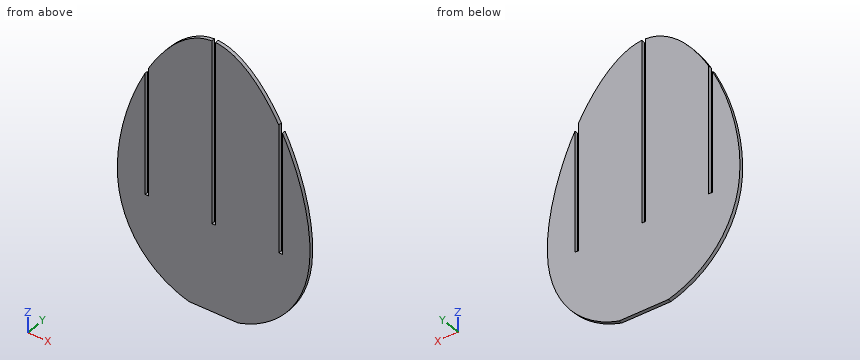
```python
from build123d import *

# Parameters (mm, degrees)
F1_DEPTH = 3


# Not quite as in the source:
# - a feature names something its author has since deleted; it is built from what else it names


with BuildPart() as f1:
    # F0 (on Front) → F1 (new body)
    with BuildSketch(Plane.XZ):
        with BuildLine():
            Line((-95.6991912493, -140.1659290001), (-95.6991912493, 9.7979199733))
            add(Edge.make_bspline(
                [(-95.6991912493, 9.7979199733), (-114.9403248651, 8.8727934734), (-134.0676037648, -9.7150772734), (-148.6991912496, -35.2231978093)],
                knots=[0.0032045269, 0.0032045269, 0.0032045269, 0.0032045269, 0.1265346274, 0.1265346274, 0.1265346274, 0.1265346274], degree=3))
            Line((-148.6991912496, -35.2231978093), (-148.6991912415, -140.1659290001))
            Line((-148.6991912415, -140.1659290001), (-151.6991912415, -140.1659290001))
            Line((-151.6991912415, -140.1659290001), (-151.6991912492, -40.6684138407))
            add(Edge.make_bspline(
                [(-151.6991912492, -40.6684138407), (-167.8134864464, -71.1210787155), (-189.9683027369, -159.0658708259), (-144.3602498784, -204.2889070632), (-114.8366912492, -212.3738275092)],
                knots=[0.135152904, 0.135152904, 0.135152904, 0.135152904, 0.2772924741, 0.4585993514, 0.4585993514, 0.4585993514, 0.4585993514], degree=3))
            Line((-114.8366912492, -212.3738275092), (-73.5616912492, -212.3738275092))
            add(Edge.make_bspline(
                [(-73.5616912492, -212.3738275092), (-44.03813262, -204.2889070632), (1.5699202449, -159.0658708196), (-20.5848960581, -71.1210786912), (-36.6991912644, -40.6684138119)],
                knots=[0.5414006486, 0.5414006486, 0.5414006486, 0.5414006486, 0.7227075259, 0.8648470961, 0.8648470961, 0.8648470961, 0.8648470961], degree=3))
            Line((-36.6991912644, -40.6684138119), (-36.6991912645, -140.1659290001))
            Line((-36.6991912645, -140.1659290001), (-39.6991912645, -140.1659290001))
            Line((-39.6991912645, -140.1659290001), (-39.6991912644, -35.223197782))
            add(Edge.make_bspline(
                [(-39.6991912644, -35.223197782), (-54.3307787472, -9.71507726), (-73.4580576403, 8.8727934739), (-92.6991912493, 9.7979199734)],
                knots=[0.8734653727, 0.8734653727, 0.8734653727, 0.8734653727, 0.9967954731, 0.9967954731, 0.9967954731, 0.9967954731], degree=3))
            Line((-92.6991912493, 9.7979199734), (-92.6991912493, -140.1659290001))
            Line((-92.6991912493, -140.1659290001), (-95.6991912493, -140.1659290001))
        make_face()
    extrude(amount=F1_DEPTH)


solid = f1.part
```
Source: CAD feature listing. Evaluate the final solid. Frame: model axes, mm. Coordinates: 2 decimals unless noted, no trailing zeros. Write each loop counter-clockwise with the first axis right and the second up, starting at its lowest first coordinate (ties: lowest second). Pieces come first, ordered by that corner, then holes. Notation, with made-up numbers: (70, 85.5) - (80, 85.5) arc R21 cw to (80, 115.5) - close; hole circle Ø1 at (-23.75, 51). An arc over 180 degrees is marked (long way). Answer as a JSON object with one key per item and string values.
Q1. Section query A-A, the plane z = -38. Output: boundary loops of the cut face in (x, y), plus the area to 3 significant figures.
Ans:
{"outline": "(-148.7, -3) - (-95.7, -3) - (-95.7, 0) - (-148.7, 0) - close; (-92.7, -3) - (-39.7, -3) - (-39.7, 0) - (-92.7, 0) - close", "area": "318 mm2"}
Q2. Section query B-B, the plane z = -113. State how many separate pieces and enclosed holes the cut face has, plus the area to 3 significant figures.
Ans:
{"separate pieces": "4", "enclosed holes": "0", "area": "452 mm2"}
Q3. First-contact query: pin 1 Ø1.5 at (y, z) = (-1.5, -113) entering from -X; pin 2 Ø1 at (y, z) = (-2, -131) entering from +X; pin 3 Ø0.9 at (y, z) = (-2, -67.5) entering from +X. Flat tips, straight axial feed; report the tip coordinate or a pass-through.
Ans:
{"pin 1": "stops at x = -174.15", "pin 2": "stops at x = -13.57", "pin 3": "stops at x = -24.76"}
Q4. Material intervals for line 1 (X direction, y = -0.7, z = -55); line 2 (X direction, y = -1.7, z = -117); line 3 (X direction, y = -0.4, z = -29), sorted ascending. Write a range as [from, to].
Ans:
{"line 1": "x = [-158.55, -151.7], [-148.7, -95.7], [-92.7, -39.7], [-36.7, -29.84]", "line 2": "x = [-174.44, -151.7], [-148.7, -95.7], [-92.7, -39.7], [-36.7, -13.96]", "line 3": "x = [-144.95, -95.7], [-92.7, -43.45]"}
